CAD build for the part. Positions are in the model's coordinates, mm. A direction names the side the tool comes from. Give positions to 0.01 mm unless a question says otherwise; leave off trailing zeros. Order: outer loops, then holes, each group sorted by start corner. A loop starts at its lowest first (then second) coordinate and runs counter-clockwise, first axis right, second up. Notation, with made-up numbers: (15.25, 35) -> (29.25, 35) arc R31 ccw to (29.25, 63) -> close; hole circle Ø7 at (20, 89). An arc over 180 degrees is marked (long way). Answer as CSV lines item,"result".
```python
from build123d import *

# Parameters (mm, degrees)
SKETCH1_R           = 1.6
BOSS_EXTRUDE1_DEPTH = 2
FILLET1_R           = 5


with BuildPart() as part:
    # Sketch1 → Boss-Extrude1 (new body)
    with BuildSketch(Plane.XY):
        Polygon((-22.25, 0), (22.25, 0), (22.25, 14.5), (7.25, 14.5), (7.25, 44.5), (-7.25, 44.5), (-7.25, 14.5), (-22.25, 14.5), align=None)
        with Locations((0, 7.25)):
            Circle(SKETCH1_R, mode=Mode.SUBTRACT)
        with Locations((15, 7.25)):
            Circle(SKETCH1_R, mode=Mode.SUBTRACT)
        with Locations((0, 22.25)):
            Circle(SKETCH1_R, mode=Mode.SUBTRACT)
        with Locations((0, 37.25)):
            Circle(SKETCH1_R, mode=Mode.SUBTRACT)
        with Locations((-15, 7.25)):
            Circle(SKETCH1_R, mode=Mode.SUBTRACT)
    extrude(amount=BOSS_EXTRUDE1_DEPTH)

    # Fillet1
    fillet1_edges = [part.edges().sort_by_distance(p)[0] for p in [
        (22.25, 14.5, 1),
        (22.25, 0, 1),
        (-22.25, 0, 1),
        (-22.25, 14.5, 1),
        (-7.25, 14.5, 1),
        (-7.25, 44.5, 1),
        (7.25, 44.5, 1),
        (7.25, 14.5, 1),
    ]]
    fillet(fillet1_edges, radius=FILLET1_R)


solid = part.part
```
1) Band-saw the part on A-A, the plane x = 15. Write the cut outline in (y, z).
Data:
outline,"(0, 0) -> (5.65, 0) -> (5.65, 2) -> (0, 2) -> close; (8.85, 0) -> (14.5, 0) -> (14.5, 2) -> (8.85, 2) -> close"
2) Band-saw the part on D-D, the plane y = 7.25. Write the cut outline in (x, z).
Data:
outline,"(-22.25, 0) -> (-16.6, 0) -> (-16.6, 2) -> (-22.25, 2) -> close; (-13.4, 0) -> (-1.6, 0) -> (-1.6, 2) -> (-13.4, 2) -> close; (1.6, 0) -> (13.4, 0) -> (13.4, 2) -> (1.6, 2) -> close; (16.6, 0) -> (22.25, 0) -> (22.25, 2) -> (16.6, 2) -> close"
3) Band-saw the part on B-B, the plane z = 0.55. Write the cut outline in (x, y), then the cut area to 3 significant figures.
Data:
outline,"(-22.25, 5) arc R5 ccw to (-17.25, 0) -> (17.25, 0) arc R5 ccw to (22.25, 5) -> (22.25, 9.5) arc R5 ccw to (17.25, 14.5) -> (12.25, 14.5) arc R5 cw to (7.25, 19.5) -> (7.25, 39.5) arc R5 ccw to (2.25, 44.5) -> (-2.25, 44.5) arc R5 ccw to (-7.25, 39.5) -> (-7.25, 19.5) arc R5 cw to (-12.25, 14.5) -> (-17.25, 14.5) arc R5 ccw to (-22.25, 9.5) -> close; hole circle Ø3.2 at (-15, 7.25); hole circle Ø3.2 at (0, 7.25); hole circle Ø3.2 at (0, 22.25); hole circle Ø3.2 at (0, 37.25); hole circle Ø3.2 at (15, 7.25)"
area,"1,020 mm2"
4) Pin check, flat tips, straight feed: P1, Ø5, axis at x = 15, y = 7.25, coming from the +Z side; P2, Ø1, axis at y = 23, z = 1, coming from the +X side; P3, Ø0.6, axis at x = -15, z = 0.5, coming from the +Y side; P4, Ø0.6, axis at y = 34.5, z = 1, coming from the -X side. Stop position of each tip, or through.
Data:
P1,"stops at z = 2"
P2,"stops at x = 7.25"
P3,"stops at y = 14.5"
P4,"stops at x = -7.25"
5) Pull direction Y, two halves, no side cores. Call faces 3 (the flat face through (0, 0, 1)), 4 (the cylindrical face through (-0.35, 5.69, 0.99)), 5 (the cylindrical face through (-16, 6, 1)), 6 (the flat face through (7.25, 29, 1)): pulls with the +Y half, pulls with the -Y half, needs draft (parallel to the pull), parting line crosses it, or undercut.
Data:
face 3,"pulls with the -Y half"
face 4,"undercut"
face 5,"undercut"
face 6,"needs draft"
6) Which spindle directions (+Z, -Z, +X, -X, +Y, -Y) get a long thin tool onto all of the face, cutting with end or side? Do faces 1 (the flat face through (-15, 14.5, 1)), 2 (the cylindrical face through (14, 6, 1)). Say none if no direction does.
Data:
face 1,"+Z, -Z, -X, +Y"
face 2,"+Z, -Z"
7) Band-saw the part on C-C, the plane y = 22.25. Write the cut outline in (x, z).
Data:
outline,"(-7.25, 0) -> (-1.6, 0) -> (-1.6, 2) -> (-7.25, 2) -> close; (1.6, 0) -> (7.25, 0) -> (7.25, 2) -> (1.6, 2) -> close"
8) Wall check: line 1 along Y through (x, z) = (0, 0.5); line 2 along Y through (x, z) = (-15, 0.5); line 3 along X through (y, z) = (25, 1.25). Give the ranges that are in metal, low to high. Write a range as [from, to].
Data:
line 1,"y = [0, 5.65], [8.85, 20.65], [23.85, 35.65], [38.85, 44.5]"
line 2,"y = [0, 5.65], [8.85, 14.5]"
line 3,"x = [-7.25, 7.25]"
